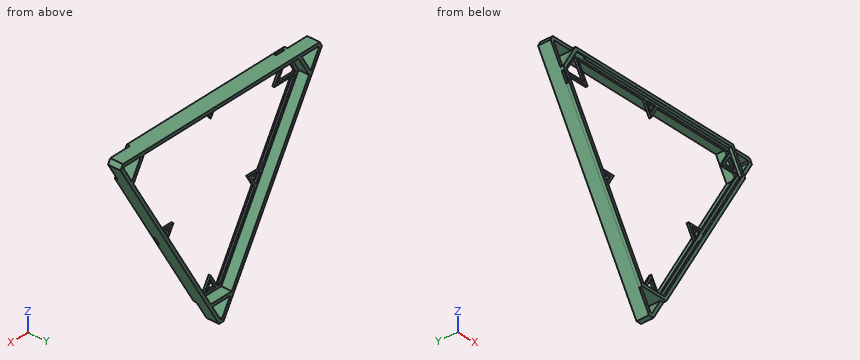
```python
from build123d import *

# Parameters (mm, degrees)
BOSS_EXTRUDE1_DEPTH = 12.38
BOSS_EXTRUDE2_DEPTH = 2
BOSS_EXTRUDE3_DEPTH = 3
SKETCH4_W           = 10
SKETCH4_H           = 2
CUT_EXTRUDE1_DEPTH  = 6
SKETCH5_W           = 10
SKETCH5_H           = 2
CUT_EXTRUDE2_DEPTH  = 6
SKETCH6_W           = 10
SKETCH6_H           = 2
CUT_EXTRUDE3_DEPTH  = 6


with BuildPart() as part:
    # Sketch1 → Boss-Extrude1 (new body)
    with BuildSketch(Plane(origin=(0, 0, 0), x_dir=(1, 0, 0), z_dir=(0, 1, 0))):
        Polygon((109.556624327, -4.42820323), (-109.556624327, -4.42820323), (-112.113248654, 0), (-2.55662435, 189.757639654), (2.556624303, 189.757639654), (112.113248654, 0), align=None)
        Polygon((-107.82457352, -1.42820323), (-108.649147039, 0), (-99.473720558, 15.892304845), (-89.473720559, -1.42820323), align=None, mode=Mode.SUBTRACT)
        Polygon((-0.824573543, 186.757639627), (0.824573481, 186.757639627), (9.999999979, 170.86533478), (-10.000000021, 170.86533478), align=None, mode=Mode.SUBTRACT)
        Polygon((108.649147039, 0), (107.82457353, -1.428203222), (89.473720569, -1.428203222), (99.473720569, 15.892304853), align=None, mode=Mode.SUBTRACT)
        Polygon((-11.732050803, 167.865334802), (11.732050803, 167.865334802), (97.741669765, 18.89230486), (86.00961895, -1.428203229), (-86.009618944, -1.428203229), (-97.741669751, 18.892304845), align=None, mode=Mode.SUBTRACT)
    extrude(amount=BOSS_EXTRUDE1_DEPTH)

    # Sketch1<4> → Boss-Extrude2 (add)
    with BuildSketch(Plane(origin=(0, 0, 0), x_dir=(1, 0, 0), z_dir=(0, 1, 0))):
        Polygon((11.732050803, 167.865334802), (-11.732050803, 167.865334802), (-97.741669751, 18.892304845), (-86.009618944, -1.428203229), (86.00961895, -1.428203229), (97.741669765, 18.89230486), align=None)
        Polygon((-84.566243256, 1.071796796), (-94.854918378, 18.892304849), (-74.277568135, 18.892304849), align=None, mode=Mode.SUBTRACT)
        Polygon((-1e-08, 9.732050841), (4.99999999, 1.071796803), (-5.00000001, 1.071796803), align=None, mode=Mode.SUBTRACT)
        Polygon((-45.071796745, 87.798692801), (-55.071796745, 87.798692801), (-50.071796745, 96.458946839), align=None, mode=Mode.SUBTRACT)
        Polygon((82.210580848, 14.312177834), (92.210580848, 14.312177834), (87.210580848, 5.651923796), align=None, mode=Mode.SUBTRACT)
        Polygon((48.91709624, 98.458946834), (41.607695163, 85.798692796), (56.226497316, 85.798692796), (94.854918412, 18.892304841), (93.36528139, 16.312177834), (78.746479233, 16.312177834), (86.055880312, 3.651923793), (84.566243293, 1.071796793), (7.309401088, 1.071796793), (2e-09, 13.732050847), (-7.309401083, 1.071796796), (-82.256842179, 1.071796796), (-70.813466519, 20.892304849), (-93.70021784, 20.892304849), (-56.226497283, 85.798692801), (-41.60769513, 85.798692801), (-48.917096207, 98.458946839), (-10.288675112, 165.365334792), (-7.309401077, 165.365334792), (0, 152.705080754), (7.309401077, 165.365334792), (10.288675142, 165.365334792), align=None, mode=Mode.SUBTRACT)
        Polygon((45.071796778, 87.798692803), (50.071796778, 96.458946841), (55.071796778, 87.798692803), align=None, mode=Mode.SUBTRACT)
        Polygon((0, 156.705080761), (-5, 165.365334799), (5, 165.365334799), align=None, mode=Mode.SUBTRACT)
    extrude(amount=BOSS_EXTRUDE2_DEPTH)

    # Sketch2 → Boss-Extrude3 (add)
    with BuildSketch(Plane.XZ):
        Polygon((101.205771363, -18.892304847), (87.741669751, 4.42820323), (-87.741669751, 4.42820323), (-101.205771368, -18.892304847), (-13.464101652, -170.86533478), (13.464101609, -170.86533478), align=None)
        Polygon((-11.732050819, -167.865334802), (11.732050795, -167.865334802), (97.741669739, -18.892304852), (86.009618931, 1.42820323), (-86.009618931, 1.42820323), (-97.741669763, -18.892304852), align=None, mode=Mode.SUBTRACT)
    extrude(amount=BOSS_EXTRUDE3_DEPTH)

    # Sketch4 → Cut-Extrude1 (cut)
    with BuildSketch(Plane.XY.offset(4.42820323)):
        with Locations((-79.741669751, -1)):
            Rectangle(SKETCH4_W, SKETCH4_H)
    extrude(amount=-CUT_EXTRUDE1_DEPTH, mode=Mode.SUBTRACT)

    # Sketch5 → Cut-Extrude2 (cut)
    with BuildSketch(Plane(origin=(-84.084936503, 0, -48.546460711), x_dir=(-0.4999999998935114, 0, 0.86602540384592), z_dir=(-0.86602540384592, 0, -0.4999999998935114))):
        with Locations((26.241669739, -1)):
            Rectangle(SKETCH5_W, SKETCH5_H)
    extrude(amount=-CUT_EXTRUDE2_DEPTH, mode=Mode.SUBTRACT)

    # Sketch6 → Cut-Extrude3 (cut)
    with BuildSketch(Plane(origin=(84.084936484, 0, -48.546460721), x_dir=(-0.5000000000540236, 0, -0.8660254037532481), z_dir=(0.8660254037532481, 0, -0.5000000000540236))):
        with Locations((53.499999991, -1)):
            Rectangle(SKETCH6_W, SKETCH6_H)
    extrude(amount=-CUT_EXTRUDE3_DEPTH, mode=Mode.SUBTRACT)


solid = part.part
```
The model under review builds one solid part; all positions refer to its coordinate system, in mm. Coordinates: 2 decimals unless noted, no trailing zeros. Write each loop counter-clockwise with the first axis right and the second up, starting at its lowest first coordinate (ties: lowest second). Pieces come first, ordered by that corner, then holes. Notation, with made-up numbers: (-11, 13) - (18, 13) arc R9 ccw to (18, 19) - close; hole circle Ø6 at (62, 28.5). An arc over 180 degrees is marked (long way). Write item = value, one per line.
(1) For line 1 (Z direction, x = 0, y = 4.5); line 2 (Z direction, x = -9, y = 11); line 3 (X direction, y = 1.25, z = -173.5), list the stretches that pass through material, from the lowest coordinate up. Write a range as [from, to].
Result sheet:
line_1 = [-189.76, -186.76], [-170.87, -167.87], [1.43, 4.43]
line_2 = [-178.6, -172.6], [-170.87, -167.87], [1.43, 4.43]
line_3 = [-11.94, -8.48], [8.48, 11.94]
(2) Consider section A-A, the plane y = 9.75. Give the boundary of the cut face in (x, z).
Result sheet:
outline = (-112.11, 0) - (-2.56, -189.76) - (2.56, -189.76) - (112.11, 0) - (109.56, 4.43) - (-109.56, 4.43) - close; hole (-108.65, 0) - (-99.47, -15.89) - (-89.47, 1.43) - (-107.82, 1.43) - close; hole (-97.74, -18.89) - (-11.73, -167.87) - (11.73, -167.87) - (97.74, -18.89) - (86.01, 1.43) - (-86.01, 1.43) - close; hole (-10, -170.87) - (-0.82, -186.76) - (0.82, -186.76) - (10, -170.87) - close; hole (89.47, 1.43) - (99.47, -15.89) - (108.65, 0) - (107.82, 1.43) - close
(3) Consider section C-C, the plane z = -80. Give the boundary of the cut face in (x, y), then the cut area to 3 significant figures.
Result sheet:
outline = (-65.93, -3) - (-62.46, -3) - (-62.46, 0) - (-59.57, 0) - (-59.57, 2) - (-62.46, 2) - (-62.46, 12.38) - (-65.93, 12.38) - close; (59.57, 0) - (62.46, 0) - (62.46, -3) - (65.93, -3) - (65.93, 12.38) - (62.46, 12.38) - (62.46, 2) - (59.57, 2) - close
area = 118 mm^2
(4) For P1, Ø2.5, axis at x = -41, y = -1, coming from the -Z side; P2, Ø1.5, axis at y = 5.5, z = -107, coming from the -X side; P3, Ø4, axis at x = 56.5, y = 4, coming from the -Z side, all flat-tipped, find the tip position at first contact; note any pin that passes through.
Result sheet:
P1 = -125.34
P2 = -50.77
P3 = -99.79
(5) Consider section B-B, the plane x = 17.5. Give the boundary of the cut face in (y, z), then the cut area to 3 significant figures.
Result sheet:
outline = (-3, -163.87) - (12.38, -163.87) - (12.38, -157.87) - (2, -157.87) - (2, -152.87) - (0, -152.87) - (0, -157.87) - (-3, -157.87) - close; (-3, 1.43) - (0, 1.43) - (0, -1.07) - (2, -1.07) - (2, 1.43) - (12.38, 1.43) - (12.38, 4.43) - (-3, 4.43) - close
area = 153 mm^2
